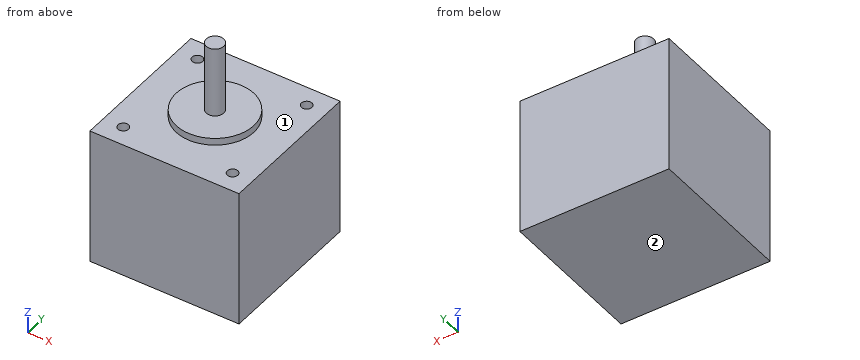
from build123d import *

# Parameters (mm, degrees)
SKIZZE1_W                       = 42.3
SKIZZE1_H                       = 42.3
AUFSATZ_LINEAR_AUSTRAGEN1_DEPTH = 39
SKIZZE2_R                       = 11
AUFSATZ_LINEAR_AUSTRAGEN2_DEPTH = 2
SKIZZE3_R                       = 2.5
AUFSATZ_LINEAR_AUSTRAGEN3_DEPTH = 20
SKIZZE4_R                       = 1.5
SCHNITT_LINEAR_AUSTRAGEN1_DEPTH = 4


with BuildPart() as part:
    # Skizze1 → Aufsatz-Linear austragen1 (new body)
    with BuildSketch(Plane.XY):
        Rectangle(SKIZZE1_W, SKIZZE1_H)
    extrude(amount=AUFSATZ_LINEAR_AUSTRAGEN1_DEPTH)

    # Skizze2 → Aufsatz-Linear austragen2 (add)
    with BuildSketch(Plane.XY.offset(39)):
        Circle(SKIZZE2_R)
    extrude(amount=AUFSATZ_LINEAR_AUSTRAGEN2_DEPTH)

    # Skizze3 → Aufsatz-Linear austragen3 (add)
    with BuildSketch(Plane.XY.offset(41)):
        Circle(SKIZZE3_R)
    extrude(amount=AUFSATZ_LINEAR_AUSTRAGEN3_DEPTH)

    # Skizze4 → Schnitt-Linear austragen1 (cut)
    with BuildSketch(Plane.XY.offset(39)):
        with Locations((-15.5, 15.5)):
            Circle(SKIZZE4_R)
        with Locations((15.5, 15.5)):
            Circle(SKIZZE4_R)
        with Locations((15.5, -15.5)):
            Circle(SKIZZE4_R)
        with Locations((-15.5, -15.5)):
            Circle(SKIZZE4_R)
    extrude(amount=-SCHNITT_LINEAR_AUSTRAGEN1_DEPTH, mode=Mode.SUBTRACT)


solid = part.part
Source: CAD feature listing. Evaluate the final solid. Frame: model axes, mm. Face numbers are marked on the shaded views. A direction names the side the tool comes from. Coordinates: 2 decimals unless noted, no trailing zeros. Loops run counter-clockwise (first coordinate to the right, second up) from the corner with the lowest first, then second, coordinate; pieces in that order, holes last. Notation, with made-up numbers: (-7, 42) - (52, 42) arc R37 cw to (52, 81) - close; hole circle Ø2 at (46, 16). An arc over 180 degrees is marked (long way). One line per item, written item: value. Start each with the question number.
1. Section C-C (x = 5). Return the cut outline in (y, z), and give its area (3 significant figures).
2. Contact query for flat-ended pins moving along their axis: P1, Ø8, axis at x = 2.5, y = -13.5, coming from the -Z side; P2, Ø3.5, axis at x = -15.5, y = -15, coming from the +Z side; P3, Ø2.5, axis at x = 15.5, y = -15.5, coming from the +Z side. Output: stop coordinate, or through.
3. Section A-A (x = 15.5). Return the cut outline in (y, z).
4. Set-up query: the marked faces 1 and 2. Return all of +Z, -Z, +X, -X, +Y, -Y with unobstructed straight access to the full face (end or side cutting, diameter ignored); none if empty.
5. Ray query, L1, parallel to Y at x = 15.5, z = 37.3; L2, parallel to Z at x = 17.5, y = 12.5; L3, parallel to X at y = 15, z = 36. Return the intervals inside material, ascending.
Verdict:
1. outline: (-21.15, 0) - (21.15, 0) - (21.15, 39) - (9.8, 39) - (9.8, 41) - (-9.8, 41) - (-9.8, 39) - (-21.15, 39) - close
1. area: 1,690 mm2
2. P1: stops at z = 0
2. P2: stops at z = 39
2. P3: stops at z = 35
3. outline: (-21.15, 0) - (21.15, 0) - (21.15, 39) - (17, 39) - (17, 35) - (14, 35) - (14, 39) - (-14, 39) - (-14, 35) - (-17, 35) - (-17, 39) - (-21.15, 39) - close
4. face 1: +Z
4. face 2: -Z, +X, -X, +Y, -Y
5. L1: y = -21.15 to -17, -14 to 14, 17 to 21.15
5. L2: z = 0 to 39
5. L3: x = -21.15 to -16.91, -14.09 to 14.09, 16.91 to 21.15
